Design review of the part shown in the three views and the two pictorial views. Dimensions are in mm from the part's minimum x, y and z. Round coordinates to 2 decimals unless told otherwise and drop trailing zeros. Order: outer loops, then holes, each group sorted by start corner. A loop starts at its lowest first (then second) coordinate and runs counter-clockwise, first axis right, second up.
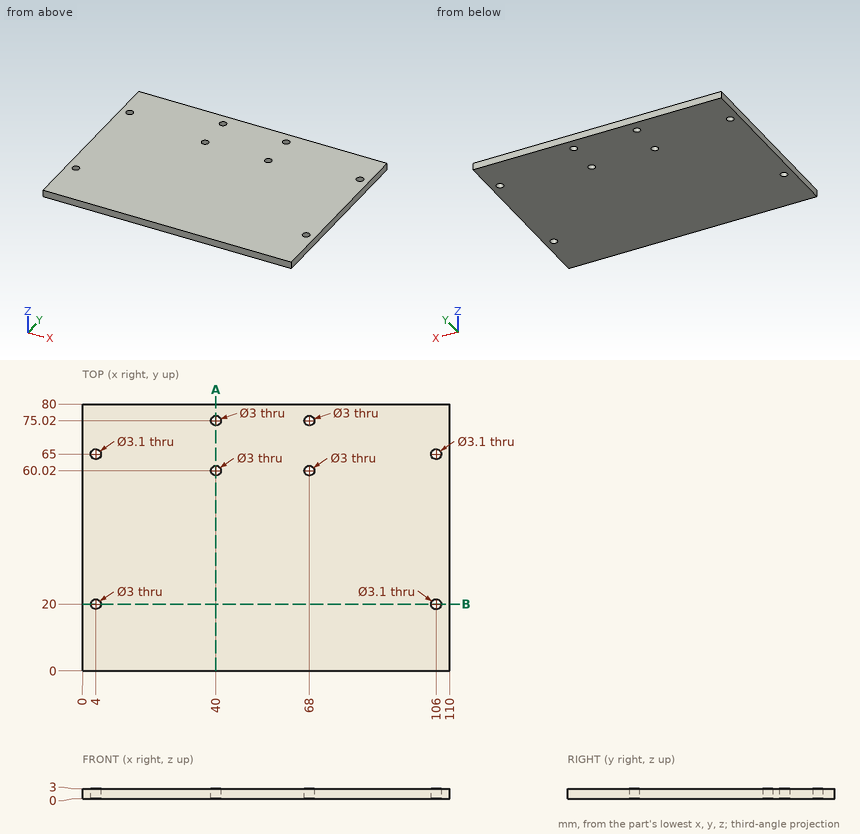
(1) Consider section B-B (y = 20). Write out the cut boundary in (x, z).
Data:
outline: (0, 0) - (2.5, 0) - (2.5, 3) - (0, 3) - close; (5.5, 0) - (104.45, 0) - (104.45, 3) - (5.5, 3) - close; (107.55, 0) - (110, 0) - (110, 3) - (107.55, 3) - close
(2) Insertion check: pin 1 (5 mm diameter, centred on x = 106, y = 20, fed in from -Z); pin 2 (1.8 mm diameter, centred on x = 40, y = 75.02, fed in from +Z). Each pin has a flat end and moves straight along its axis. Give the tip position at first contact, or say it passes through.
Data:
pin 1: stops at z = 0
pin 2: passes through
(3) To check wall thickness, follow probe 1 along Y at (x, z) = (4, 2.1); probe 2 along Y at (x, z) = (68, 1.8). State the ranges of each line that lie inside material, in increasing order.
Data:
probe 1: y = 0 to 18.5, 21.5 to 63.45, 66.55 to 80
probe 2: y = 0 to 58.52, 61.52 to 73.52, 76.52 to 80
(4) Consider section A-A (x = 40). Write out the cut boundary in (y, z), and give its area (3 significant figures).
Data:
outline: (0, 0) - (58.52, 0) - (58.52, 3) - (0, 3) - close; (61.52, 0) - (73.52, 0) - (73.52, 3) - (61.52, 3) - close; (76.52, 0) - (80, 0) - (80, 3) - (76.52, 3) - close
area: 222 mm2
